Design review of the part shown in the three views and the two pictorial views. Dimensions are in mm from the part's minimum x, y and z. Coordinates: 2 decimals unless noted, no trailing zeros. Write each loop counter-clockwise with the first axis right and the second up, starting at its lowest first coordinate (ties: lowest second). Pieces come first, ordered by that corner, then holes. Notation, with made-up numbers: (52, 10.5) - (58, 10.5) arc R25 ccw to (58, 37.5) - close; hole circle Ø5 at (68.5, 71.5). An arc over 180 degrees is marked (long way). Return JSON: item names as keys, results as strings. Group by question number.
(1) We need section B-B on x = 36.83. State the section outline as (y, z) points.
(2) For pin 1 Ø3 at (x, y) = (77.47, 17.78) entering from -Z, flat-tipped, find the tip position at first contact; note if it passes through.
(3) We need section A-A on z = 3.5. Give the number of separate pieces and of enclosed holes in the cut face, then the cut area to 3 significant figures.
(4) We need section C-C on y = 11. State the section outline as (x, z) points (3 decimals), then the cut area to 3 significant figures.
(5) We need section D-D on y = 60.5. State the section outline as (x, z) points, then the cut area to 3 significant figures.
(6) To check wall thickness, follow L1, parallel to X at y = 119, z = 4.75; L2, parallel to X at y = 18.5, z = 3.5; L3, parallel to X at y = 40, z = 5. State the ranges of each line that lie inside material, in increasing order. Write a range as from..to.
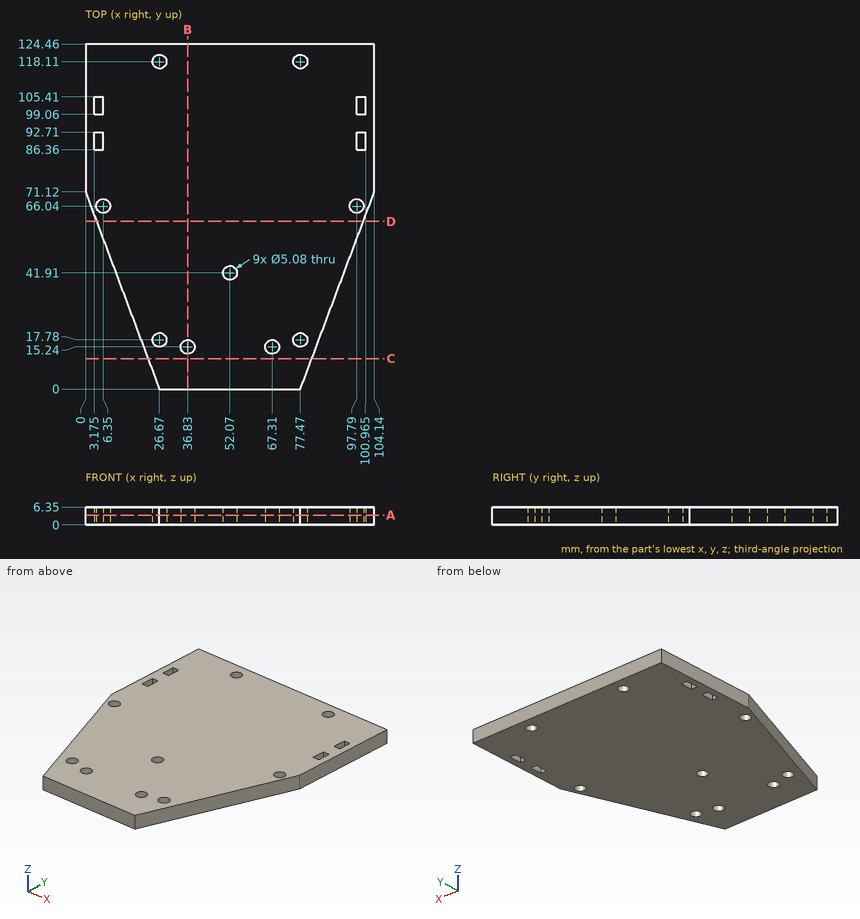
Ans:
{
 "1": {"outline": "(0, 0) - (12.7, 0) - (12.7, 6.35) - (0, 6.35) - close; (17.78, 0) - (124.46, 0) - (124.46, 6.35) - (17.78, 6.35) - close"},
 "2": {"pin 1": "through"},
 "3": {"separate pieces": "1", "enclosed holes": "13", "area": "10,800 mm²"},
 "4": {"outline": "(22.545, 0) - (81.595, 0) - (81.595, 6.35) - (22.545, 6.35) - close", "area": "375 mm²"},
 "5": {"outline": "(3.98, 0) - (100.16, 0) - (100.16, 6.35) - (3.98, 6.35) - close", "area": "611 mm²"},
 "6": {"L1": "0..24.29, 29.05..75.09, 79.85..104.14", "L2": "19.73..24.23, 29.11..75.03, 79.91..84.41", "L3": "11.67..50.4, 53.74..92.47"}
}
